Part print with two shaded views. Sizes in mm from the minimum x, y, z corner. Round coordinates to 2 decimals unless told otherwise and drop trailing zeros. Loops run counter-clockwise (first coordinate to the right, second up) from the corner with the lowest first, then second, coordinate; pieces in that order, holes last. Notation, with made-up numbers: (-21.5, -21.75) - (20.5, -21.75) arc R19 cw to (20.5, 11.25) - close; hole circle Ø10 at (72.25, 32). An arc over 180 degrees is marked (long way). Use a Markdown table: item, result.
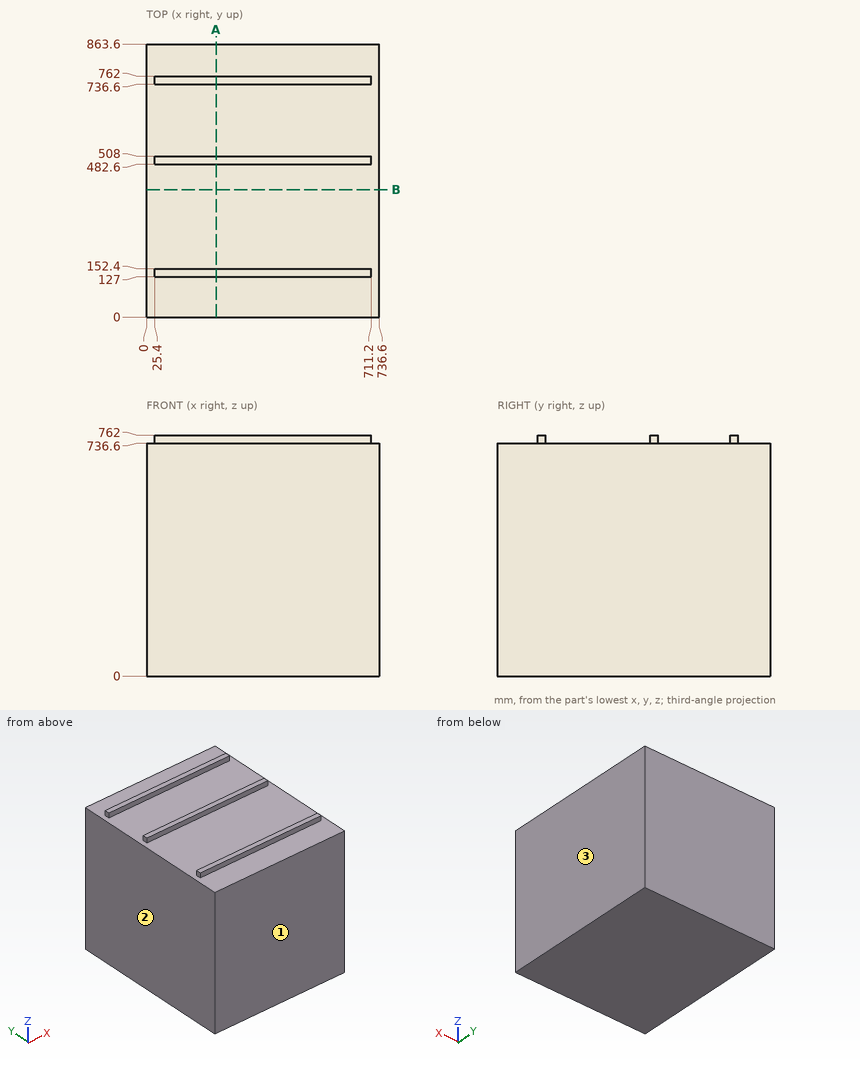
Q1. Cut at A-A, the plane x = 220.5. List the corners of the cut face in (y, z), plus the area to 3 significant figures.
Results found:
| item | result |
|---|---|
| outline | (0, 0) - (863.6, 0) - (863.6, 736.6) - (762, 736.6) - (762, 762) - (736.6, 762) - (736.6, 736.6) - (508, 736.6) - (508, 762) - (482.6, 762) - (482.6, 736.6) - (152.4, 736.6) - (152.4, 762) - (127, 762) - (127, 736.6) - (0, 736.6) - close |
| area | 638,000 mm2 |
Q2. Pull direction X, two halves, no side cores. Call the marked faces 1, 2 and 3: pulls with the +X half, pulls with the -X half, needs draft (parallel to the pull), parting line crosses it, or undercut.
Results found:
| item | result |
|---|---|
| face 1 | needs draft |
| face 2 | pulls with the -X half |
| face 3 | pulls with the +X half |
Q3. Drop flat-ended pins along their axis: pin 1 (5 mm diameter, centred on y = 261.5, z = 323.5, fed in from -X); pin 2 (20.5 mm diameter, centred on x = 221, z = 751.5, fed in from +Y); pin 3 (20.5 mm diameter, centred on y = 745.5, z = 751.5, fed in from -X); pin 4 (12.5 mm diameter, centred on y = 747.5, z = 745, fed in from +X). Give the stop position or say it passes through.
Results found:
| item | result |
|---|---|
| pin 1 | stops at x = 0 |
| pin 2 | stops at y = 762 |
| pin 3 | stops at x = 25.4 |
| pin 4 | stops at x = 711.2 |
Q4. Cut at B-B, the plane y = 403. List the corners of the cut face in (x, z), plus the area to 3 significant figures.
Results found:
| item | result |
|---|---|
| outline | (0, 0) - (736.6, 0) - (736.6, 736.6) - (0, 736.6) - close |
| area | 543,000 mm2 |
Q5. Probe line 1 (Z direction, x = 640.5, y = 229.5). List the from-to ranges inside material, lowest first.
Results found:
| item | result |
|---|---|
| line 1 | z = 0 to 736.6 |
